Print and shaded views of the part. All mm, measured from the part's lowest x, y and z. A direction names the side the tool comes from. Coordinates: 2 decimals unless noted, no trailing zeros. Order: outer loops, then holes, each group sorted by start corner. A loop starts at its lowest first (then second) coordinate and runs counter-clockwise, first axis right, second up. Notation, with made-up numbers: (52.5, -4) - (80.5, -4) arc R22 ccw to (80.5, 5) - close; hole circle Ø1 at (8.5, 20.25). An arc over 180 degrees is marked (long way). Write each question's results on one line, items separated by ' | '.
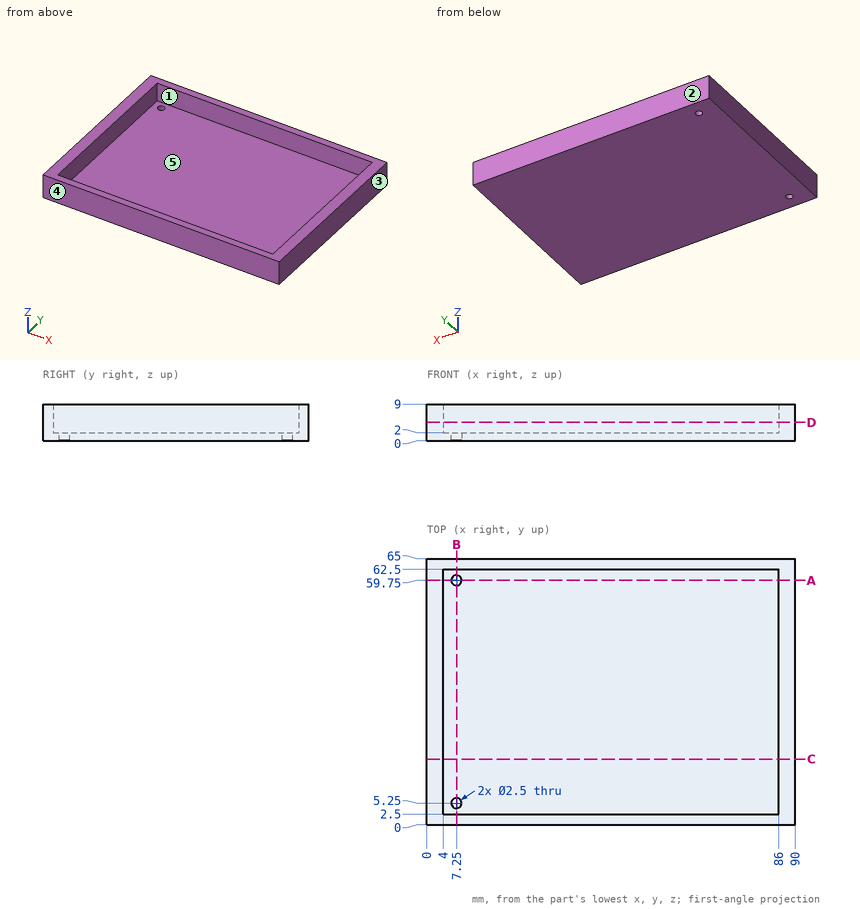
1. Band-saw the part on A-A on y = 59.75. Give the cut face in (x, z), then the cut area to 3 significant figures.
Solved:
outline: (0, 0) - (6, 0) - (6, 2) - (4, 2) - (4, 9) - (0, 9) - close; (8.5, 0) - (90, 0) - (90, 9) - (86, 9) - (86, 2) - (8.5, 2) - close | area: 231 mm2
2. Band-saw the part on B-B on x = 7.25. Give the cut face in (y, z).
Solved:
outline: (0, 0) - (4, 0) - (4, 2) - (2.5, 2) - (2.5, 9) - (0, 9) - close; (6.5, 0) - (58.5, 0) - (58.5, 2) - (6.5, 2) - close; (61, 0) - (65, 0) - (65, 9) - (62.5, 9) - (62.5, 2) - (61, 2) - close
3. Tool access for the marked faces 1 and 2: list every direction of +Z, -Z, +X, -X, +Y, -Y with a clear straight run to the whole face (end or side of a thin tool).
Solved:
face 1: +Z | face 2: +Z, -Z, +X, -X, +Y
4. Band-saw the part on D-D on z = 4.5. Give the cut face in (x, y), then the cut area to 3 significant figures.
Solved:
outline: (0, 0) - (90, 0) - (90, 65) - (0, 65) - close; hole (4, 2.5) - (86, 2.5) - (86, 62.5) - (4, 62.5) - close | area: 930 mm2
5. Two-plate mould, pull along X, no slides. Class the marked faces 3, 4 and 5: +X half, -X half, draft (parallel to the pull), parting line (faces both ways), or undercut.
Solved:
face 3: +X half | face 4: draft | face 5: undercut
6. Band-saw the part on C-C on y = 16. Give the cut face in (x, z), then the cut area to 3 significant figures.
Solved:
outline: (0, 0) - (90, 0) - (90, 9) - (86, 9) - (86, 2) - (4, 2) - (4, 9) - (0, 9) - close | area: 236 mm2
7. Drop a flat-ended pin along its axis: pin 1 Ø4 at (y, z) = (12.5, 6.5) entering from -X. Give the stop position or say it passes through.
Solved:
pin 1: stops at x = 0
8. Probe line 1 (Y direction, x = 7.25, z = 1.25); line 2 (X direction, y = 9.5, z = 7.25); line 3 (Y direction, x = 74.5, z = 2.25). List the from-to ranges inside material, lowest first.
Solved:
line 1: y = 0 to 4, 6.5 to 58.5, 61 to 65 | line 2: x = 0 to 4, 86 to 90 | line 3: y = 0 to 2.5, 62.5 to 65
